Part print with two shaded views. Sizes in mm from the minimum x, y, z corner. Round coordinates to 2 decimals unless told otherwise and drop trailing zeros. Write each loop counter-clockwise with the first axis right and the second up, starting at its lowest first coordinate (ties: lowest second). Pieces come first, ordered by that corner, then holes. Notation, with made-up numbers: M -1,28.5 L 30,28.5 A12 ccw 30,34.5 Z; hole C -36.5,-2 d2. An arc over 180 degrees is marked long. One line per question, with ' | ' between items. Start each with the question number.
1) Saw through at A-A (y = 7.5). List the corners of the cut face in (x, z).
2) Saw through at C-C (z = 3). Give the number of separate pieces and of enclosed holes in the cut face, plus the area to 3 significant figures.
3) Wall check: probe 1 along X at (y, z) = (132.7, 5); probe 2 along Y at (x, z) = (112.5, 6.75); probe 3 along X at (y, z) = (112.5, 3.75). Give the ranges that are in metal, low to high. Write a range as [from, to].
4) Saw through at B-B (x = 7.5). List the corners of the cut face in (y, z).
5) Drop a flat-ended pin along its axis: pin 1 Ø4.5 at (x, z) = (72.5, 5.5) entering from +Y. Give the stop position or say it passes through.
6) Saw through at D-D (x = 21). List the corners of the cut face in (y, z).
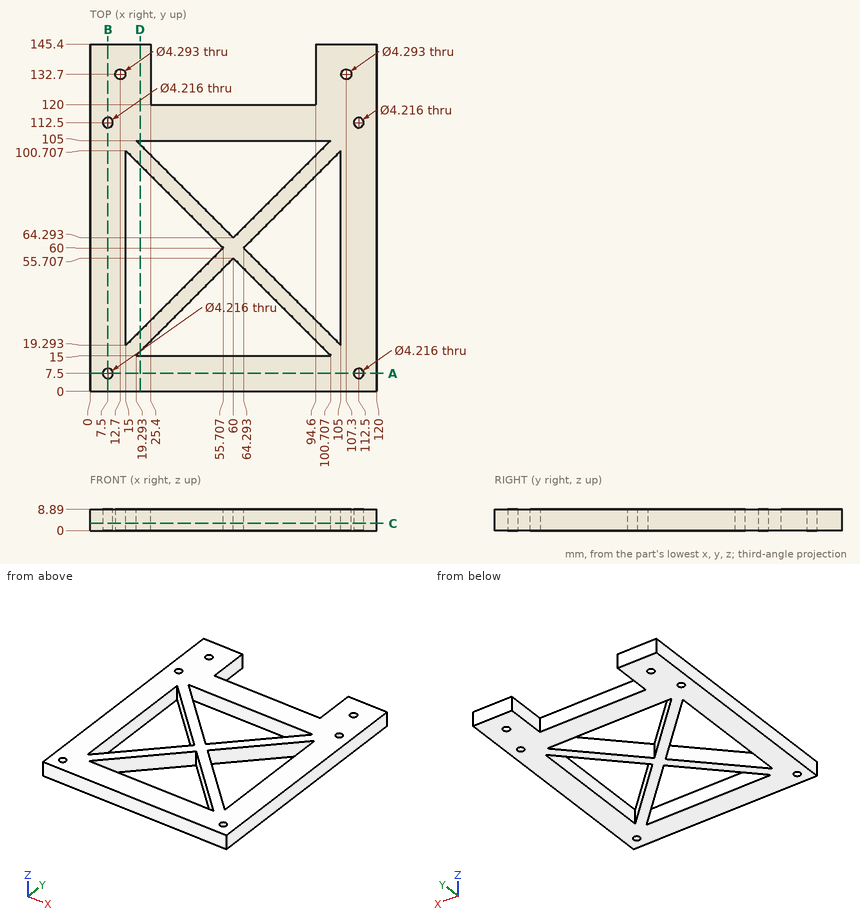
Answer key:
1) outline: M 0,0 L 5.39,0 L 5.39,8.89 L 0,8.89 Z; M 9.61,0 L 110.39,0 L 110.39,8.89 L 9.61,8.89 Z; M 114.61,0 L 120,0 L 120,8.89 L 114.61,8.89 Z
2) separate pieces: 1 | enclosed holes: 10 | area: 8,980 mm2
3) probe 1: x = [0, 10.55], [14.85, 25.4], [94.6, 105.15], [109.45, 120] | probe 2: y = [0, 5.39], [9.61, 110.39], [114.61, 145.4] | probe 3: x = [0, 5.39], [9.61, 110.39], [114.61, 120]
4) outline: M 0,0 L 5.39,0 L 5.39,8.89 L 0,8.89 Z; M 9.61,0 L 110.39,0 L 110.39,8.89 L 9.61,8.89 Z; M 114.61,0 L 145.4,0 L 145.4,8.89 L 114.61,8.89 Z
5) pin 1: stops at y = 120
6) outline: M 0,0 L 15,0 L 15,8.89 L 0,8.89 Z; M 16.71,0 L 25.29,0 L 25.29,8.89 L 16.71,8.89 Z; M 94.71,0 L 103.29,0 L 103.29,8.89 L 94.71,8.89 Z; M 105,0 L 145.4,0 L 145.4,8.89 L 105,8.89 Z
